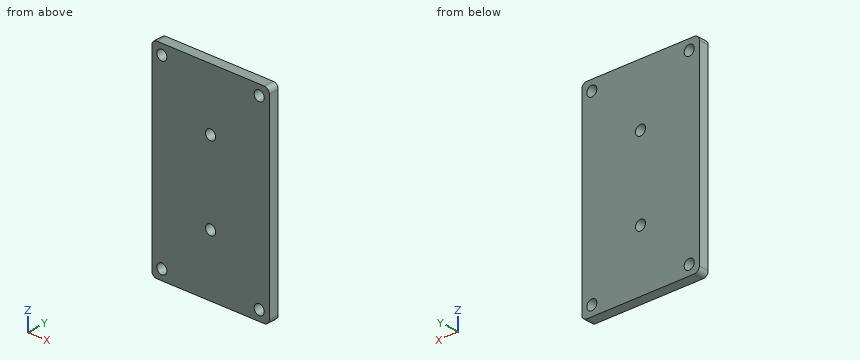
Autodesk Inventor part; units mm, degrees
ref_plane "YZ Plane" through (0, 0, 0) normal (1, 0, 0) x (0, 1, 0)
ref_plane "XZ Plane" through (0, 0, 0) normal (0, 1, 0) x (-1, 0, 0)
ref_plane "XY Plane" through (0, 0, 0) normal (0, 0, 1) x (1, 0, 0)
sketch "Sketch1" plane through (0, 0, 0) normal (0, 1, 0) x (-1, 0, 0)
  line L0 (11.5, 24) -> (-11.5, 24)
  line L1 (-11.5, 24) -> (-11.5, -24)
  line L2 (-11.5, -24) -> (11.5, -24)
  line L3 (11.5, -24) -> (11.5, 24)
  line L4 (11.5, 24) -> (-11.5, -24) construction
  line L5 (-11.5, 24) -> (11.5, -24) construction
  line L6 (-8.5, 21) -> (8.5, 21)
  line L7 (8.5, 21) -> (8.5, -21)
  line L8 (8.5, -21) -> (-8.5, -21)
  line L9 (-8.5, -21) -> (-8.5, 21)
  line L10 (-8.5, 21) -> (8.5, -21) construction
  line L11 (8.5, 21) -> (-8.5, -21) construction
  line L12 (0, 0) -> (-8.5, 0) construction
  circle A0 centre (0, -12) radius 1.5
  circle A1 centre (0, 12) radius 1.5
  line L13 (17.5, 30) -> (-17.5, 30)
  line L14 (-17.5, 30) -> (-17.5, -30)
  line L15 (-17.5, -30) -> (17.5, -30)
  line L16 (17.5, -30) -> (17.5, 30)
  line L17 (17.5, 30) -> (-17.5, -30) construction
  line L18 (-17.5, 30) -> (17.5, -30) construction
  circle A2 centre (14.5, 27) radius 1.5
  circle A3 centre (-14.5, 27) radius 1.5
  circle A4 centre (14.5, -27) radius 1.5
  circle A5 centre (-14.5, -27) radius 1.5
  dimension "d0" = 23
  dimension "d1" = 48
  dimension "d3" = 3
  dimension "d4" = 3
  dimension "d5" = 3
  dimension "d6" = 12
  dimension "d9" = 6
  dimension "d10" = 6
  dimension "d13" = 3
  dimension "d14" = 3
  dimension "d15" = 3
  dimension "d16" = 3
  dimension "d17" = 3
  dimension "d18" = 3
extrude "Extrusion1" add sketch "Sketch1" along normal blind 3 contours L3 L2 L1 L0 | L6 L7 L8 L9 | L16 L15 L14 L13
fillet "Fillet2" radius 1.5 4 edges at (17.5, 1.5, -30) (17.5, 1.5, 30) (-17.5, 1.5, 30) (-17.5, 1.5, -30)
properties part number "Top&Bottom"
For this review, take the finished solid that the model builds, in its own axes (mm). Coordinates: 2 decimals unless noted, no trailing zeros. Loops run counter-clockwise (first coordinate to the right, second up) from the corner with the lowest first, then second, coordinate; pieces in that order, holes last. Notation, with made-up numbers: (87, 49.5) - (123, 49.5) arc R21 cw to (123, 55.5) - close; hole circle Ø9 at (17, 57). An arc over 180 degrees is marked (long way). Use one line per item in the form item = value. Start each with the question number.
1) Take a section at B-B (x = -14.5). State the section outline as (y, z) points.
2) Take a section at C-C (y = 2). State the section outline as (x, z) points, plus the area to 3 significant figures.
3) Take a section at A-A (z = 27). State the section outline as (x, y) points.
4) To check wall thickness, follow probe 1 along Z at (x, y) = (14.5, 2.4); probe 2 along Z at (x, y) = (0, 2.1); probe 3 along X at (y, z) = (0.7, -11.5). State the ranges of each line that lie inside material, in increasing order. Write a range as from..to.
5) For pin 1 (2.5 mm diameter, centred on x = 14.5, z = 27, fed in from -Y), flat-tipped, find the tip position at first contact; note if it passes through.
From the geometry:
q1.outline = (0, -30) - (3, -30) - (3, -28.5) - (0, -28.5) - close; (0, -25.5) - (3, -25.5) - (3, 25.5) - (0, 25.5) - close; (0, 28.5) - (3, 28.5) - (3, 30) - (0, 30) - close
q2.outline = (-17.5, -28.5) arc R1.5 ccw to (-16, -30) - (16, -30) arc R1.5 ccw to (17.5, -28.5) - (17.5, 28.5) arc R1.5 ccw to (16, 30) - (-16, 30) arc R1.5 ccw to (-17.5, 28.5) - close; hole circle Ø3 at (-14.5, -27); hole circle Ø3 at (-14.5, 27); hole circle Ø3 at (0, -12); hole circle Ø3 at (0, 12); hole circle Ø3 at (14.5, -27); hole circle Ø3 at (14.5, 27)
q2.area = 2,060 mm2
q3.outline = (-17.5, 0) - (-16, 0) - (-16, 3) - (-17.5, 3) - close; (-13, 0) - (13, 0) - (13, 3) - (-13, 3) - close; (16, 0) - (17.5, 0) - (17.5, 3) - (16, 3) - close
q4.probe_1 = -30..-28.5, -25.5..25.5, 28.5..30
q4.probe_2 = -30..-13.5, -10.5..10.5, 13.5..30
q4.probe_3 = -17.5..-1.41, 1.41..17.5
q5.pin_1 = through
